Input: part model. Units: mm. Frame: model coordinates. A direction names the side the tool comes from. Round coordinates to 2 decimals unless told otherwise and drop trailing zeros. Order: outer loops, then holes, each group sorted by start corner. A loop starts at its lowest first (then second) coordinate and runs counter-clockwise, first axis right, second up. Notation, with made-up numbers: (33.25, -19.75) -> (48.25, -19.75) arc R21 ccw to (48.25, 17.25) -> close; hole circle Ø5 at (29, 0). An arc over 180 degrees is marked (long way). Answer as CSV lines item,"result". Start each with the question number.
1) Access query for faces 4 (the face through (30, 17, -3)), 5 (the face through (42.81, 38.52, -8.54)), 6 (the face through (13.785, 23.974, -48.521)). Directions: +Z, -Z, +X, -X, +Y, -Y. A direction counts if a zero-diameter tool reaches every point of the face in a straight line with its end or side. Return the directions, or none.
2) Section query D-D, the plane z = -9.5. Output: boundary loops of the cut face in (x, y), and give its area (3 significant figures).
3) Mould query, pull axis X, two halves, no side actions, for faces 1 (the face through (60, 38, -21)), 2 (the face through (15.523, 5.088, -48.521)), 3 (the face through (29.58, 39.43, -0.6)). Classes: +X half, -X half, draft (parallel to the pull), parting line (faces both ways), or undercut.
4) Line query: L1, parallel to Z at x = 48, y = 3; L2, parallel to Y at x = 7, z = -44; L3, parallel to X at y = 38, z = -40. Output: solid intervals per line, ascending.
5) First-contact query: P1, Ø4, axis at x = 13.5, z = -27, coming from the -Y side; P2, Ø3, axis at x = 30.475, y = 5, coming from the -Z side. Flat tips, straight axial feed; report the tip coordinate or a pass-through.
6) Section query B-B, the plane y = 33.5. Output: boundary loops of the cut face in (x, z), and give its area (3 significant figures).
7) Section query A-A, the plane x = 8. Output: boundary loops of the cut face in (y, z).
8) Section query C-C, the plane z = -25. Output: boundary loops of the cut face in (x, y).
```python
from build123d import *

# Parameters (mm, degrees)
EXTRUDE_1_DEPTH     = 60
CUT_EXTRUDE_1_REACH = 42
SKETCH_2_R          = 2.5
SKETCH_2_R_2        = 12
SKETCH_3_R          = 7
CUT_EXTRUDE_2_DEPTH = 51
CUT_EXTRUDE_3_REACH = 52
SKETCH_6_R          = 2


with BuildPart() as part:
    # 草图1 → 凸台-拉伸1 (new body)
    with BuildSketch(Plane(origin=(0, 0, 0), x_dir=(0, 0, -1), z_dir=(1, 0, 0))):
        with BuildLine():
            Line((0, 0), (3, 0))
            Line((3, 0), (3, 35))
            ThreePointArc((3, 35), (3.585786438, 36.414213562), (5, 37))
            Line((5, 37), (45, 37))
            ThreePointArc((45, 37), (46.414213562, 36.414213562), (47, 35))
            Line((47, 35), (47, 0))
            Line((47, 0), (50, 0))
            Line((50, 0), (50, 38))
            ThreePointArc((50, 38), (49.414213562, 39.414213562), (48, 40))
            Line((48, 40), (2, 40))
            ThreePointArc((2, 40), (0.585786438, 39.414213562), (0, 38))
            Line((0, 38), (0, 0))
        make_face()
    extrude(amount=EXTRUDE_1_DEPTH)

    # 草图2 → 切除-拉伸1 (cut, up to next)
    with BuildSketch(Plane(origin=(0, 40, 0), x_dir=(1, 0, 0), z_dir=(0, 1, 0)), mode=Mode.PRIVATE) as cut_extrude_1_sk1:
        with Locations((9.5, 9.5)):
            Circle(SKETCH_2_R)
    cut_extrude_1_tool1 = extrude(cut_extrude_1_sk1.sketch, amount=-CUT_EXTRUDE_1_REACH, mode=Mode.PRIVATE) & part.part
    add(cut_extrude_1_tool1.solids().sort_by_distance((9.5, 40, -9.5))[0], mode=Mode.SUBTRACT)
    # 草图2 → 切除-拉伸1 (cut, up to next)
    with BuildSketch(Plane(origin=(0, 40, 0), x_dir=(1, 0, 0), z_dir=(0, 1, 0)), mode=Mode.PRIVATE) as cut_extrude_1_sk2:
        with Locations((40.5, 9.5)):
            Circle(SKETCH_2_R)
    cut_extrude_1_tool2 = extrude(cut_extrude_1_sk2.sketch, amount=-CUT_EXTRUDE_1_REACH, mode=Mode.PRIVATE) & part.part
    add(cut_extrude_1_tool2.solids().sort_by_distance((40.5, 40, -9.5))[0], mode=Mode.SUBTRACT)
    # 草图2 → 切除-拉伸1 (cut, up to next)
    with BuildSketch(Plane(origin=(0, 40, 0), x_dir=(1, 0, 0), z_dir=(0, 1, 0)), mode=Mode.PRIVATE) as cut_extrude_1_sk3:
        with Locations((40.5, 40.5)):
            Circle(SKETCH_2_R)
    cut_extrude_1_tool3 = extrude(cut_extrude_1_sk3.sketch, amount=-CUT_EXTRUDE_1_REACH, mode=Mode.PRIVATE) & part.part
    add(cut_extrude_1_tool3.solids().sort_by_distance((40.5, 40, -40.5))[0], mode=Mode.SUBTRACT)
    # 草图2 → 切除-拉伸1 (cut, up to next)
    with BuildSketch(Plane(origin=(0, 40, 0), x_dir=(1, 0, 0), z_dir=(0, 1, 0)), mode=Mode.PRIVATE) as cut_extrude_1_sk4:
        with Locations((9.5, 40.5)):
            Circle(SKETCH_2_R)
    cut_extrude_1_tool4 = extrude(cut_extrude_1_sk4.sketch, amount=-CUT_EXTRUDE_1_REACH, mode=Mode.PRIVATE) & part.part
    add(cut_extrude_1_tool4.solids().sort_by_distance((9.5, 40, -40.5))[0], mode=Mode.SUBTRACT)
    # 草图2 → 切除-拉伸1 (cut, up to next)
    with BuildSketch(Plane(origin=(0, 40, 0), x_dir=(1, 0, 0), z_dir=(0, 1, 0)), mode=Mode.PRIVATE) as cut_extrude_1_sk5:
        with Locations((25, 25)):
            Circle(SKETCH_2_R_2)
    cut_extrude_1_tool5 = extrude(cut_extrude_1_sk5.sketch, amount=-CUT_EXTRUDE_1_REACH, mode=Mode.PRIVATE) & part.part
    add(cut_extrude_1_tool5.solids().sort_by_distance((25, 40, -25))[0], mode=Mode.SUBTRACT)

    # 草图3 → 切除-拉伸2 (cut, through all)
    with BuildSketch(Plane.XY):
        with Locations((43, 15)):
            Circle(SKETCH_3_R)
    extrude(amount=-CUT_EXTRUDE_2_DEPTH, mode=Mode.SUBTRACT)

    # 草图6 → 切除-拉伸3 (cut, up to next)
    with BuildSketch(Plane(origin=(0, 0, -50), x_dir=(-1, 0, 0), z_dir=(0, 0, -1)), mode=Mode.PRIVATE) as cut_extrude_3_sk1:
        with Locations((-13.525, 5)):
            Circle(SKETCH_6_R)
    cut_extrude_3_tool1 = extrude(cut_extrude_3_sk1.sketch, amount=-CUT_EXTRUDE_3_REACH, mode=Mode.PRIVATE) & part.part
    add(cut_extrude_3_tool1.solids().sort_by_distance((13.525, 5, -50))[0], mode=Mode.SUBTRACT)
    # 草图6 → 切除-拉伸3 (cut, up to next)
    with BuildSketch(Plane(origin=(0, 0, -50), x_dir=(-1, 0, 0), z_dir=(0, 0, -1)), mode=Mode.PRIVATE) as cut_extrude_3_sk2:
        with Locations((-30.475, 5)):
            Circle(SKETCH_6_R)
    cut_extrude_3_tool2 = extrude(cut_extrude_3_sk2.sketch, amount=-CUT_EXTRUDE_3_REACH, mode=Mode.PRIVATE) & part.part
    add(cut_extrude_3_tool2.solids().sort_by_distance((30.475, 5, -50))[0], mode=Mode.SUBTRACT)
    # 草图6 → 切除-拉伸3 (cut, up to next)
    with BuildSketch(Plane(origin=(0, 0, -50), x_dir=(-1, 0, 0), z_dir=(0, 0, -1)), mode=Mode.PRIVATE) as cut_extrude_3_sk3:
        with Locations((-30.475, 21.991100612)):
            Circle(SKETCH_6_R)
    cut_extrude_3_tool3 = extrude(cut_extrude_3_sk3.sketch, amount=-CUT_EXTRUDE_3_REACH, mode=Mode.PRIVATE) & part.part
    add(cut_extrude_3_tool3.solids().sort_by_distance((30.475, 21.991101, -50))[0], mode=Mode.SUBTRACT)
    # 草图6 → 切除-拉伸3 (cut, up to next)
    with BuildSketch(Plane(origin=(0, 0, -50), x_dir=(-1, 0, 0), z_dir=(0, 0, -1)), mode=Mode.PRIVATE) as cut_extrude_3_sk4:
        with Locations((-13.525, 21.991100612)):
            Circle(SKETCH_6_R)
    cut_extrude_3_tool4 = extrude(cut_extrude_3_sk4.sketch, amount=-CUT_EXTRUDE_3_REACH, mode=Mode.PRIVATE) & part.part
    add(cut_extrude_3_tool4.solids().sort_by_distance((13.525, 21.991101, -50))[0], mode=Mode.SUBTRACT)


solid = part.part
```
Findings:
1,face 4,"+X, -X, -Y"
1,face 5,"+Y, -Y"
1,face 6,"-Z"
2,outline,"(0, 37) -> (7, 37) -> (7, 40) -> (0, 40) -> close; (12, 37) -> (38, 37) -> (38, 40) -> (12, 40) -> close; (43, 37) -> (60, 37) -> (60, 40) -> (43, 40) -> close"
2,area,"150 mm^2"
3,face 1,"+X half"
3,face 2,"undercut"
3,face 3,"draft"
4,L1,"z = -50 to -47, -3 to 0"
4,L2,"y = 37 to 40"
4,L3,"x = 0 to 7.05, 11.95 to 38.05, 42.95 to 60"
5,P1,"stops at y = 37"
5,P2,"stops at z = -3"
6,outline,"(0, -50) -> (60, -50) -> (60, -47) -> (0, -47) -> close; (0, -3) -> (60, -3) -> (60, 0) -> (0, 0) -> close"
6,area,"360 mm^2"
7,outline,"(0, -50) -> (38, -50) arc R2 ccw to (40, -48) -> (40, -42.5) -> (37, -42.5) -> (37, -45) arc R2 cw to (35, -47) -> (0, -47) -> close; (0, -3) -> (35, -3) arc R2 cw to (37, -5) -> (37, -7.5) -> (40, -7.5) -> (40, -2) arc R2 ccw to (38, 0) -> (0, 0) -> close; (37, -38.5) -> (40, -38.5) -> (40, -11.5) -> (37, -11.5) -> close"
8,outline,"(0, 37) -> (13, 37) -> (13, 40) -> (0, 40) -> close; (37, 37) -> (60, 37) -> (60, 40) -> (37, 40) -> close"
